Design review of the part shown in the three views and the two pictorial views. Dimensions are in mm from the part's minimum x, y and z. Coordinates: 2 decimals unless noted, no trailing zeros. Loops run counter-clockwise (first coordinate to the right, second up) from the corner with the lowest first, then second, coordinate; pieces in that order, holes last. Notation, with made-up numbers: (-18, 31.25) -> (7, 31.25) arc R30 cw to (7, 66.25) -> close; hole circle Ø1 at (-32.75, 16). An arc over 180 degrees is marked (long way). Answer in a Markdown table with one row per item.
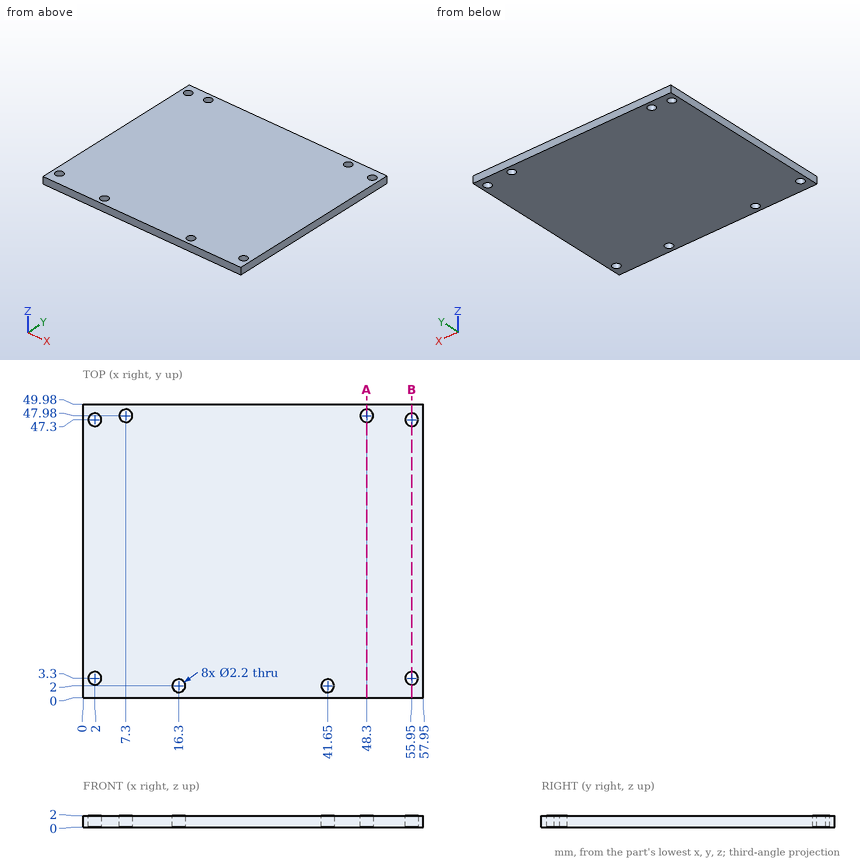
Item 1: For L1, parallel to Y at x = 7.3, z = 1.6; L2, parallel to Y at x = 49, z = 1.5, list the stretches that pass through material, from the lowest coordinate up.
Worked answers:
| item | result |
|---|---|
| L1 | 0 to 46.88, 49.08 to 49.98 |
| L2 | 0 to 47.13, 48.83 to 49.98 |
Item 2: Insertion check: pin 1 (1.3 mm diameter, centred on x = 16.3, y = 2, fed in from -Z). The pin has a flat end and moves straight along its axis. Give the tip position at first contact, or say it passes through.
Worked answers:
| item | result |
|---|---|
| pin 1 | through |
Item 3: Take a section at A-A, the plane x = 48.3. State the section outline as (y, z) points, and give its area (3 significant figures).
Worked answers:
| item | result |
|---|---|
| outline | (0, 0) -> (46.88, 0) -> (46.88, 2) -> (0, 2) -> close; (49.08, 0) -> (49.98, 0) -> (49.98, 2) -> (49.08, 2) -> close |
| area | 95.6 mm² |
Item 4: Take a section at B-B, the plane x = 55.95. State the section outline as (y, z) points, and give its area (3 significant figures).
Worked answers:
| item | result |
|---|---|
| outline | (0, 0) -> (2.2, 0) -> (2.2, 2) -> (0, 2) -> close; (4.4, 0) -> (46.2, 0) -> (46.2, 2) -> (4.4, 2) -> close; (48.4, 0) -> (49.98, 0) -> (49.98, 2) -> (48.4, 2) -> close |
| area | 91.2 mm² |
